The model under review builds one solid part; all positions refer to its coordinate system, in mm. Face numbers are marked on the shaded views. A direction names the side the tool comes from. Round coordinates to 2 decimals unless told otherwise and drop trailing zeros. Order: outer loops, then holes, each group sorted by start corner. A loop starts at its lowest first (then second) coordinate and runs counter-clockwise, first axis right, second up.
1) Consider section C-C (x = 15). Give the boundary of the cut face in (y, z), then the cut area to 3 significant figures.
2) Consider section A-A (y = 20). Give the boundary of the cut face in (x, z), then the cut area to 3 significant figures.
3) Consider section B-B (z = 1.55). Give the boundary of the cut face in (x, y).
4) To check wall thickness, follow L1, parallel to X at y = 20, z = 1.55; L2, parallel to Y at x = 17, z = 1.9; L3, parallel to X at y = 14.5, z = 3.45. State the ranges of each line that lie inside material, in increasing order.
5) Mouldability with a two-part tool opening along Y and no side actions: class the marked faces 3, 4 and 5 as pulls with the +Y half, pulls with the -Y half, needs draft (parallel to the pull), parting line crosses it, or undercut.
6) Machinability: for the marked faces 1 and 2, which of the approach directions +Z, -Z, +X, -X, +Y, -Y give a long, thin tool a straight path to every point of the face, cutting with its end or side? Answer none if there is none.
7) Consider section D-D (x = 21.75). Give the boundary of the cut face in (y, z).
8) Clearance check with flat-ended pins moving along their axes: P1, Ø8, axis at x = 11.5, y = 12, coming from the -Z side; P2, Ø10, axis at x = 13, y = 17.5, coming from the +Z side. State where each tip first meets the part, or that it passes through.
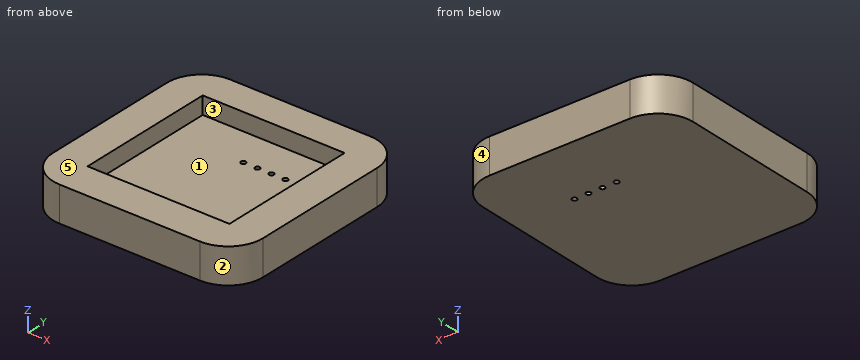
from build123d import *

# Parameters (mm, degrees)
F0_W     = 30
F0_H     = 30
F0_R     = 0.35
F1_DEPTH = 2.5
F2_W     = 30
F2_H     = 30
F2_W_2   = 20.25
F2_H_2   = 20.25
F3_DEPTH = 5
F4_R     = 5


with BuildPart() as f1:
    # F0 (on Top) → F1 (new body)
    with BuildSketch(Plane.XY):
        with Locations((15, 15)):
            Rectangle(F0_W, F0_H)
        with Locations((15, 20)):
            Circle(F0_R, mode=Mode.SUBTRACT)
        with Locations((17, 20)):
            Circle(F0_R, mode=Mode.SUBTRACT)
        with Locations((19, 20)):
            Circle(F0_R, mode=Mode.SUBTRACT)
        with Locations((21, 20)):
            Circle(F0_R, mode=Mode.SUBTRACT)
    extrude(amount=F1_DEPTH)

    # F2 (on Top) → F3 (join)
    with BuildSketch(Plane.XY):
        with Locations((15, 15)):
            Rectangle(F2_W, F2_H)
        with Locations((14.976355, 15.216224)):
            Rectangle(F2_W_2, F2_H_2, mode=Mode.SUBTRACT)
    extrude(amount=F3_DEPTH)

    # F4
    f4_edges = [f1.edges().sort_by_distance(p)[0] for p in [
        (0, 30, 2.5),
        (0, 0, 2.5),
        (30, 30, 2.5),
        (30, 0, 2.5),
    ]]
    fillet(f4_edges, radius=F4_R)


solid = f1.part
Answer below:
1. outline: (0, 0) - (19.65, 0) - (19.65, 2.5) - (5.09, 2.5) - (5.09, 5) - (0, 5) - close; (20.35, 0) - (30, 0) - (30, 5) - (25.34, 5) - (25.34, 2.5) - (20.35, 2.5) - close
1. area: 97.6 mm2
2. outline: (0, 0) - (14.65, 0) - (14.65, 2.5) - (4.85, 2.5) - (4.85, 5) - (0, 5) - close; (15.35, 0) - (16.65, 0) - (16.65, 2.5) - (15.35, 2.5) - close; (17.35, 0) - (18.65, 0) - (18.65, 2.5) - (17.35, 2.5) - close; (19.35, 0) - (20.65, 0) - (20.65, 2.5) - (19.35, 2.5) - close; (21.35, 0) - (30, 0) - (30, 5) - (25.1, 5) - (25.1, 2.5) - (21.35, 2.5) - close
2. area: 92.4 mm2
3. outline: (0, 5) arc R5 ccw to (5, 0) - (25, 0) arc R5 ccw to (30, 5) - (30, 25) arc R5 ccw to (25, 30) - (5, 30) arc R5 ccw to (0, 25) - close; hole circle Ø0.7 at (15, 20); hole circle Ø0.7 at (17, 20); hole circle Ø0.7 at (19, 20); hole circle Ø0.7 at (21, 20)
4. L1: x = 0 to 14.65, 15.35 to 16.65, 17.35 to 18.65, 19.35 to 20.65, 21.35 to 30
4. L2: y = 0 to 19.65, 20.35 to 30
4. L3: x = 0 to 4.85, 25.1 to 30
5. face 3: undercut
5. face 4: pulls with the +Y half
5. face 5: needs draft
6. face 1: +Z
6. face 2: +Z, -Z, +X, -Y
7. outline: (0, 0) - (30, 0) - (30, 5) - (25.34, 5) - (25.34, 2.5) - (5.09, 2.5) - (5.09, 5) - (0, 5) - close
8. P1: stops at z = 0
8. P2: stops at z = 2.5
